Source: three-view drawing plus pictorial views. Frame: mm from the lowest corner of the part. Give positions to 0.01 mm unless a question says otherwise; leave off trailing zeros. Loops run counter-clockwise (first coordinate to the right, second up) from the corner with the lowest first, then second, coordinate; pieces in that order, holes last. Notation, with made-up numbers: M 79,27.25 L 96,27.25 A16 ccw 96,41.25 Z; hole C 44,55.5 d6. An arc over 180 degrees is marked long. Answer as a JSON object with one key per item and string values. Group by question number.
1) Section query A-A on z = 43. Return loops of the section in (x, y).
2) Section query C-C on x = 23. Return loops of the section in (y, z).
3) First-contact query: P1, Ø1.6, axis at x = 7.5, y = 23.5, coming from the -Z side; P2, Ø1, axis at y = 18, z = 8, coming from the -X side; P3, Ø1.5, axis at y = 12.5, z = 36, coming from the -X side. Flat tips, straight axial feed; report the tip coordinate or a pass-through.
4) Ray query, L1, parallel to Y at x = 7, z = 7; L2, parallel to X at y = 6, z = 6.5; L3, parallel to Z at x = 21.5, y = 7. Return the intervals inside material, ascending.
5) Section query D-D on x = 28.25. Return loops of the section in (y, z).
6) Section query B-B on y = 22. Return loops of the section in (x, z), plus the area to 3 significant figures.
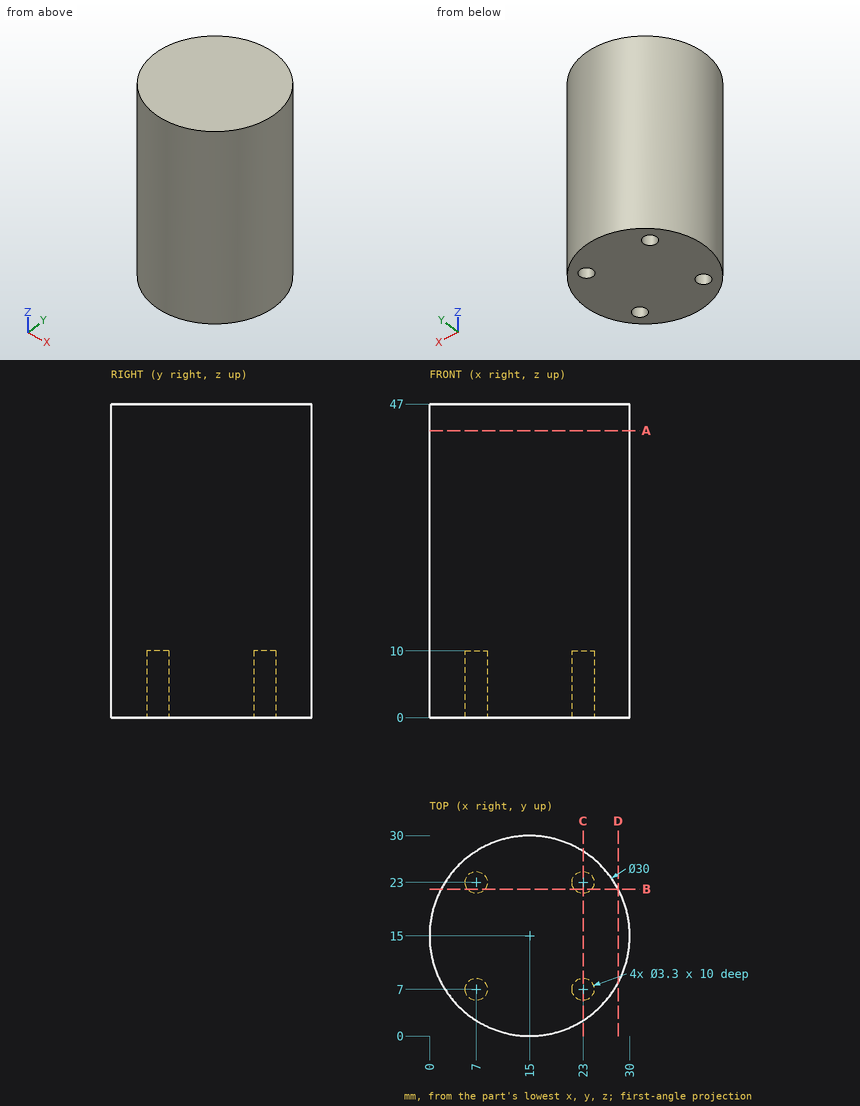
Output:
{
 "1": {"outline": "C 15,15 d30"},
 "2": {"outline": "M 2.31,0 L 5.35,0 L 5.35,10 L 8.65,10 L 8.65,0 L 21.35,0 L 21.35,10 L 24.65,10 L 24.65,0 L 27.69,0 L 27.69,47 L 2.31,47 Z"},
 "3": {"P1": "stops at z = 10", "P2": "stops at x = 0.21", "P3": "stops at x = 0.1"},
 "4": {"L1": "y = 2.31 to 5.35, 8.65 to 21.35, 24.65 to 27.69", "L2": "x = 3 to 5.69, 8.31 to 21.69, 24.31 to 27", "L3": "z = 10 to 47"},
 "5": {"outline": "M 7.97,0 L 22.03,0 L 22.03,47 L 7.97,47 Z"},
 "6": {"outline": "M 1.73,0 L 5.69,0 L 5.69,10 L 8.31,10 L 8.31,0 L 21.69,0 L 21.69,10 L 24.31,10 L 24.31,0 L 28.27,0 L 28.27,47 L 1.73,47 Z", "area": "1,190 mm^2"}
}
